Part model, mm, in its own coordinate system. A direction names the side the tool comes from. Round coordinates to 2 decimals unless told otherwise and drop trailing zeros. Write each loop counter-clockwise with the first axis right and the second up, starting at its lowest first coordinate (ties: lowest second). Pieces come first, ordered by that corner, then holes. Notation, with made-up numbers: (60, -6.75) -> (94, -6.75) arc R23 ccw to (94, 24.25) -> close; hole circle Ø8 at (89, 59.5). An arc over 180 degrees is marked (long way). Return JSON: item names as keys, results as strings. Group by question number.
(1) Saw through at B-B (x = 43.9). List the corners of the cut face in (y, z).
(2) Tool access for faces 1 (the flat face through (22, 0, -15)), 2 (the flat face through (24, 3.2, -8)), 3 (the flat face through (24, 1, -14.6)): list every direction of +Z, -Z, +X, -X, +Y, -Y with a clear straight run to the whole face (end or side of a thin tool).
(3) Saw through at A-A (y = 0.7). State how many separate pieces and enclosed holes the cut face has, plus the area to 3 significant figures.
(4) Mould opens along Z. For faces 4 (the flat face through (24, 2, -15.8)), 5 (the cylindrical face through (21.09, 2.79, -4.06)), 6 (the flat face through (12, 4.8, -4)) say: +Z half, -Z half, draft (parallel to the pull), parting line (faces both ways), or undercut.
(5) Drill centre lines: L1, parallel to Z at x = 11.9, y = 3; L2, parallel to X at y = 1.4, z = -1.25; L3, parallel to Z at x = 6, y = 0.6. Where is each one in solid material? Low to high. Write a range as from..to.
(6) Drop flat-ended pins along their axis: pin 1 Ø2.5 at (x, z) = (20, -12.5) entering from -Y; pin 2 Ø5.5 at (x, z) = (40, -8) entering from -Y; pin 3 Ø5.5 at (x, z) = (31.9, -7.9) entering from +Y. Give the stop position or say it passes through.
from build123d import *

# Parameters (mm, degrees)
SKETCH1_W            = 47.8
SKETCH1_H            = 3.2
BOSS_EXTRUDE1_DEPTH  = 15.8
SKETCH2_R            = 2.4
BOSS_EXTRUDE2_DEPTH  = 1.6
LPATTERN1_COUNT      = 2
LPATTERN1_PITCH      = 8
LPATTERN1_COUNT_DIR2 = 6
LPATTERN1_PITCH_DIR2 = 8
SHELL1_T             = -1.2
SKETCH4_R            = 3.25
SKETCH4_R_2          = 2.4
BOSS_EXTRUDE3_DEPTH  = 1.8
LPATTERN2_COUNT      = 5
LPATTERN2_PITCH      = 8


with BuildPart() as part:
    # Sketch1 → Boss-Extrude1 (new body)
    with BuildSketch(Plane.XY):
        with Locations((23.9, 1.6)):
            Rectangle(SKETCH1_W, SKETCH1_H)
    extrude(amount=-BOSS_EXTRUDE1_DEPTH)

    # Sketch2 → Boss-Extrude2 (add)
    with BuildSketch(Plane(origin=(0, 3.2, 0), x_dir=(1, 0, 0), z_dir=(0, 1, 0))):
        with Locations(Location((3.9, 3.9, 0), (0, 0, 270))):
            Circle(SKETCH2_R)
    boss_extrude2 = extrude(amount=BOSS_EXTRUDE2_DEPTH)

    # LPattern1: Boss-Extrude2 2 × 6
    with Locations(*[(j * LPATTERN1_PITCH_DIR2, 0, -i * LPATTERN1_PITCH) for i in range(LPATTERN1_COUNT) for j in range(LPATTERN1_COUNT_DIR2) if (i, j) != (0, 0)]):
        add(boss_extrude2)

    # Shell1
    shell1_openings = [part.faces().sort_by_distance(p)[0] for p in [
        (23.9, 0, -7.9),
    ]]
    offset(amount=SHELL1_T, openings=shell1_openings, kind=Kind.INTERSECTION)

    # Sketch4 → Boss-Extrude3 (add)
    with BuildSketch(Plane.XZ.offset(-2)):
        with Locations(Location((7.9, -7.9, 0), (0, 0, 90))):
            Circle(SKETCH4_R)
        with Locations(Location((7.9, -7.9, 0), (0, 0, 270))):
            Circle(SKETCH4_R_2, mode=Mode.SUBTRACT)
    boss_extrude3 = extrude(amount=BOSS_EXTRUDE3_DEPTH)

    # LPattern2: Boss-Extrude3 ×5
    with Locations(*[(i * LPATTERN2_PITCH, 0, 0) for i in range(1, LPATTERN2_COUNT)]):
        add(boss_extrude3)


solid = part.part
Computed values:
{
 "1": {"outline": "(0, -15.8) -> (3.2, -15.8) -> (3.2, -14.3) -> (4.8, -14.3) -> (4.8, -9.5) -> (3.2, -9.5) -> (3.2, -6.3) -> (4.8, -6.3) -> (4.8, -1.5) -> (3.2, -1.5) -> (3.2, 0) -> (0, 0) -> (0, -1.2) -> (2, -1.2) -> (2, -2.7) -> (3.6, -2.7) -> (3.6, -5.1) -> (2, -5.1) -> (2, -10.7) -> (3.6, -10.7) -> (3.6, -13.1) -> (2, -13.1) -> (2, -14.6) -> (0, -14.6) -> close"},
 "2": {"face 1": "+Z, -Z, +X, -X, -Y", "face 2": "+Y", "face 3": "-Y"},
 "3": {"separate pieces": "6", "enclosed holes": "6", "area": "222 mm2"},
 "4": {"face 4": "-Z half", "face 5": "undercut", "face 6": "draft"},
 "5": {"L1": "-15.8..-13.1, -10.7..-5.1, -2.7..0", "L2": "0..1.2, 46.6..47.8", "L3": "-15.8..-14.6, -10.54..-9.37, -6.43..-5.26, -1.2..0"},
 "6": {"pin 1": "y = 2", "pin 2": "y = 0.2", "pin 3": "y = 3.2"}
}
